Autodesk Inventor part; units mm, degrees
ref_plane "YZ Plane" through (0, 0, 0) normal (1, 0, 0) x (0, 1, 0)
ref_plane "XZ Plane" through (0, 0, 0) normal (0, 1, 0) x (-1, 0, 0)
ref_plane "XY Plane" through (0, 0, 0) normal (0, 0, 1) x (1, 0, 0)
sketch "Sketch1" plane through (0, 0, 0) normal (0, 1, 0) x (-1, 0, 0)
  line L0 (30, 30) -> (-30, 30)
  line L1 (-30, 30) -> (-30, -30)
  line L2 (-30, -30) -> (30, -30)
  line L3 (30, -30) -> (30, 30)
  circle A0 centre (0, 0) radius 2.0484
  dimension "d0" = 60
  dimension "d1" = 60
  dimension "d2" = 30
  dimension "d3" = 30
extrude "Extrusion1" add sketch "Sketch1" against normal blind 10
sketch "Sketch2" plane through (0, -10, 0) normal (0, -1, 0) x (1, 0, 0)
  line L0 (30, -30) -> (30, 30)
  line L1 (-30, 30) -> (-30, -30)
  line L2 (30, 30) -> (-30, 30)
  line L3 (-30, 30) -> (-30, -30)
  line L4 (-30, -30) -> (30, -30)
  line L5 (30, -30) -> (30, 30)
  line L6 (20, 20) -> (-20, 20)
  line L7 (-20, 20) -> (-20, -20)
  line L8 (-20, -20) -> (20, -20)
  line L9 (20, -20) -> (20, 20)
  point P0 (0, 0)
  dimension "d6" = 10
  dimension "d7" = 10
  dimension "d8" = 10
  dimension "d9" = 10
extrude "Extrusion2" add sketch "Sketch2" along normal blind 120
sketch "Sketch3" plane through (-30, 0, 30) normal (0, 0, 1) x (1, 0, 0)
  point P0 (30, 0)
sketch "Sketch4" plane through (-30, 0, 30) normal (0, 0, 1) x (1, 0, 0)
  line L0 (50, -10) -> (10, -10)
  line L1 (50, -10) -> (50, -130)
  line L2 (10, -10) -> (50, -10)
  line L3 (50, -10) -> (50, -95)
  line L4 (50, -95) -> (10, -95)
  line L5 (10, -95) -> (10, -10)
  point P0 (30, 0)
  dimension "d12" = 85
extrude "Extrusion3" cut sketch "Sketch4" against normal blind 10
sketch "Sketch5" plane through (-30, 0, 30) normal (0, 0, 1) x (1, 0, 0)
  line L0 (60, 0) -> (60, -130)
  line L1 (60, -130) -> (0, -130)
  line L2 (60, -95) -> (0, -95)
  line L3 (0, -95) -> (0, -130)
  line L4 (0, -130) -> (60, -130)
  line L5 (60, -130) -> (60, -95)
  point P0 (30, 0)
  dimension "d16" = 35
extrude "Extrusion4" cut sketch "Sketch5" against normal blind 30
sketch "Sketch6" plane through (-20, -10, -20) normal (0, 0, 1) x (1, 0, 0)
  line L0 (-10, -85) -> (0, -85)
  line L1 (0, -85) -> (40, -85)
  line L2 (40, -85) -> (40, -120)
  line L3 (40, -120) -> (0, -120)
  line L4 (0, -120) -> (0, -85)
  point P0 (20, 10)
extrude "Extrusion5" add sketch "Sketch6" along normal blind 20
sketch "Sketch7" plane through (-30, 0, 0) normal (0, 0, 1) x (1, 0, 0)
  circle A0 centre (10, -105) radius 1.95
  circle A1 centre (10, -120) radius 1.95
  circle A2 centre (50, -105) radius 1.95
  circle A3 centre (50, -120) radius 1.95
  line L0 (60, -95) -> (60, -130)
  line L1 (60, -130) -> (0, -130)
  line L2 (50, -95) -> (60, -95)
  line L3 (50, -95) -> (10, -95)
  line L4 (0, -130) -> (0, -95)
  point P0 (30, 0)
  dimension "d21" = 10
  dimension "d22" = 10
  dimension "d23" = 10
  dimension "d24" = 10
  dimension "d25" = 10
  dimension "d26" = 10
  dimension "d27" = 10
  dimension "d28" = 10
  dimension "d29" = 3.9
  dimension "d30" = 3.9
  dimension "d31" = 3.9
  dimension "d32" = 3.9
extrude "Extrusion6" cut sketch "Sketch7" against normal blind 35
sketch "Sketch8" plane through (30, 0, -30) normal (0, 0, -1) x (-1, 0, 0)
  circle A0 centre (10, -105) radius 1.95
  circle A1 centre (10, -105) radius 4.5
  circle A2 centre (10, -120) radius 1.95
  circle A3 centre (10, -120) radius 4.5
  circle A4 centre (50, -105) radius 1.95
  circle A5 centre (50, -105) radius 4.5
  circle A6 centre (50, -120) radius 1.95
  circle A7 centre (50, -120) radius 4.5
  point P0 (30, 0)
  dimension "d35" = 9
  dimension "d36" = 9
  dimension "d37" = 9
  dimension "d38" = 9
extrude "Extrusion7" cut sketch "Sketch8" against normal blind 15 contours A0 | A1 | A3 | A5 | A7
sketch "Sketch9" plane through (0, 0, 0) normal (0, 1, 0) x (1, 0, 0)
  circle A0 centre (0, 0) radius 6.5
  circle A1 centre (0, -7) radius 15.5
  line L0 (30, -30) -> (30, 30)
  line L1 (0, -7) -> (-17.1994, -7)
  line L2 (-17.1994, -7) -> (16.6076, -7)
  line L3 (0, -7) -> (-8.5199, -21.7569)
  line L4 (0, -7) -> (9.3939, -23.2707)
  line L5 (0, -7) -> (10.7829, 11.6765)
  line L6 (0, -7) -> (-10.6515, 11.4489)
  circle A2 centre (7.75, 6.4234) radius 1.5
  circle A3 centre (-7.75, 6.4234) radius 1.5
  circle A4 centre (-15.5, -7) radius 1.5
  circle A5 centre (-7.75, -20.4234) radius 1.5
  circle A6 centre (7.75, -20.4234) radius 1.5
  circle A7 centre (15.5, -7) radius 1.5
  dimension "d44" = 13
  dimension "d45" = 31
  dimension "d46" = 7
  dimension "d47" = 30
  dimension "d48" = 60
  dimension "d49" = 60
  dimension "d50" = 60
  dimension "d51" = 60
  dimension "d52" = 3
  dimension "d53" = 3
  dimension "d54" = 3
  dimension "d55" = 3
  dimension "d56" = 3
  dimension "d57" = 3
extrude "Extrusion8" cut sketch "Sketch9" against normal blind 10 contours A0 L5 | L5 A0 L6 | L6 A0 | A2 A1 L5 | L5 A1 A2 | A3 A1 L6 | L6 A1 A3 | L5 A2 A1 | A1 A2 L5 | A4 A1 L1 | L1 A1 A4 | A7 A1 L2 | L2 A1 A7 | A5 A1 L3 | L3 A1 A5 | A6 A1 L4 | L4 A1 A6 | L6 A3 A1 | A1 A3 L6 | A7 A1 | L1 A4 A1 | A1 A4 L1 | L3 A5 A1 | A1 A5 L3 | L4 A6 A1 | A1 A6 L4 picked at (0.3591, 1.0442)
properties part number "Base_V2c"
Input: part model. Units: mm. Frame: model coordinates. A direction names the side the tool comes from. Round coordinates to 2 decimals unless told otherwise and drop trailing zeros. Write each loop counter-clockwise with the first axis right and the second up, starting at its lowest first coordinate (ties: lowest second). Pieces come first, ordered by that corner, then holes. Notation, with made-up numbers: M 65.25,7 L 69.25,7 A9 ccw 69.25,23 Z; hole C 72.25,-4 d9. An arc over 180 degrees is marked long. Write each question's results on one line, items separated by ' | '.
Q1. Section query D-D (z = -25). Return loops of the section in (x, y).
Results:
outline: M -30,-130 L 30,-130 L 30,0 L -30,0 Z; hole C -20,-120 d9; hole C -20,-105 d9; hole C 20,-120 d9; hole C 20,-105 d9
Q2. Section query A-A (z = 2.5). Return loops of the section in (x, y).
Results:
outline: M -30,-95 L -20,-95 L -20,-10 L -6,-10 L -6,0 L -30,0 Z; M 6,-10 L 20,-10 L 20,-95 L 30,-95 L 30,0 L 6,0 Z
Q3. Line query: line 1 along X through (y, z) = (-120, -3.25); line 2 along X through (y, z) = (-3, 7); line 3 along Z through (x, y) = (-7.75, -6.25). Output: solid intervals per line, ascending.
Results:
line 1: x = -30 to -21.95, -18.05 to 18.05, 21.95 to 30 | line 2: x = -30 to -17, -14 to 14, 17 to 30 | line 3: z = -30 to -7.92, -4.92 to 18.92, 21.92 to 30
Q4. Section query B-B (x = 0). Return loops of the section in (y, z), and give its area (3 significant figures).
Results:
outline: M -130,-30 L 0,-30 L 0,-6.5 L -10,-6.5 L -10,-20 L -95,-20 L -95,0 L -130,0 Z; M -10,6.5 L 0,6.5 L 0,30 L -10,30 Z | area: 2,370 mm^2
Q5. Section query C-C (y = -105). Return loops of the section in (x, z), and give its area (3 significant figures).
Results:
outline: M -30,-30 L -24.5,-30 L -24.5,-15 L -21.95,-15 L -21.95,0 L -30,0 Z; M -18.05,-15 L -15.5,-15 L -15.5,-30 L 15.5,-30 L 15.5,-15 L 18.05,-15 L 18.05,0 L -18.05,0 Z; M 21.95,-15 L 24.5,-15 L 24.5,-30 L 30,-30 L 30,0 L 21.95,0 Z | area: 1,410 mm^2
Q6. Access query for faces 5 (the face through (-21.948, -119.914, -7.395)), 6 (the face through (-16.4, -122.7, -22.6)), 7 (the face through (-20, -52, 5)), 8 (the face through (6.56, -4.93, -5.51)). Directions: +Z, -Z, +X, -X, +Y, -Y. A direction counts if a zero-diameter tool reaches every point of the face in a straight line with its end or side. Return the directions, or none.
Results:
face 5: +Z, -Z | face 6: -Z | face 7: +Z | face 8: +Y
Q7. Pin query (flat end, axial travel): P1, Ø8, axis at x = 26.5, z = 12.5, coming from the -Y side; P2, Ø7, axis at x = 20, y = -120, coming from the -Z side; P3, Ø4, axis at x = 14.5, z = 12, coming from the -Y side; P4, Ø2.5, axis at x = 7.75, z = 20.42, coming from the +Y side. Return the tip coordinate at first contact, or that it passes through.
Results:
P1: stops at y = -95 | P2: stops at z = -15 | P3: stops at y = -10 | P4: passes through
Q8. Draft query along Z for faces 1 (the face through (-17, -5, 7)), 2 (the face through (0, -52, -20)), 3 (the face through (-22, -106, -15)), 4 (the face through (19.577, -106.904, -7.395)). Return one class per face: released by +Z, released by -Z, zero draft, split by the parting line, or undercut.
Results:
face 1: undercut | face 2: released by +Z | face 3: released by -Z | face 4: zero draft
